```python
from build123d import *

# Parameters (mm, degrees)
SKETCH1_W           = 170
SKETCH1_H           = 120
BOSS_EXTRUDE1_DEPTH = 8
SKETCH2_W           = 41.380626675
SKETCH2_H           = 10
BOSS_EXTRUDE2_DEPTH = 8
SKETCH3_R           = 2
CUT_EXTRUDE1_DEPTH  = 8


with BuildPart() as part:
    # Sketch1 → Boss-Extrude1 (new body)
    with BuildSketch(Plane(origin=(0, 0, 0), x_dir=(1, 0, 0), z_dir=(0, 1, 0))):
        Rectangle(SKETCH1_W, SKETCH1_H)
    extrude(amount=BOSS_EXTRUDE1_DEPTH)

    # Sketch2 → Boss-Extrude2 (add)
    with BuildSketch(Plane(origin=(-17.791513114, 8, -1.374929401), x_dir=(1, 0, 0), z_dir=(0, 1, 0))):
        with Locations((-32.208486886, 28.840032215)):
            Rectangle(SKETCH2_W, SKETCH2_H)
    extrude(amount=BOSS_EXTRUDE2_DEPTH)

    # Sketch3 → Cut-Extrude1 (cut)
    with BuildSketch(Plane(origin=(0, 8, 0), x_dir=(1, 0, 0), z_dir=(0, 1, 0))):
        with Locations((-80, 55)):
            Circle(SKETCH3_R)
        with Locations((-80, -55)):
            Circle(SKETCH3_R)
        with Locations((80, 55)):
            Circle(SKETCH3_R)
        with Locations((80, -55)):
            Circle(SKETCH3_R)
    extrude(amount=-CUT_EXTRUDE1_DEPTH, mode=Mode.SUBTRACT)


solid = part.part
```
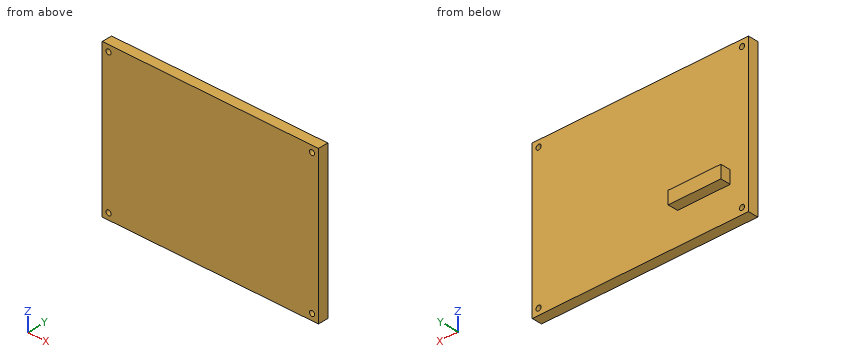
Read the model definition and answer for the solid it produces. Units are mm, in the model's axes. Give positions to 0.01 mm unless a question says otherwise; leave off trailing zeros. Write each loop counter-clockwise with the first axis right and the second up, starting at its lowest first coordinate (ties: lowest second). Pieces come first, ordered by that corner, then holes. Notation, with made-up numbers: M 66,27.25 L 95,27.25 A28 ccw 95,48.25 Z; hole C 51.5,-27.75 d2. An arc over 180 degrees is marked long. Put each result on its own line as item: value. Start each with the question number.
1. The part is cut by section D-D, the plane y = 12. Give the vertices of the cut face in (x, z).
2. The part is cut by section A-A, the plane x = -80. Give the vertices of the cut face in (y, z), and give its area (3 significant figures).
3. The part is cut by section B-B, the plane z = -55. Give the vertices of the cut face in (x, y), and give its area (3 significant figures).
4. The part is cut by section C-C, the plane x = -42.5. Give the vertices of the cut face in (y, z).
5. Consider line 1 along Z through (x, y) = (-80, 2.25); line 2 along X through (y, z) = (4.75, 55); line 3 along Y through (x, z) = (53.5, 52.5). Determine where each line is inside the solid, lowest interval first.
6. Each of these flat-tipped pins is pushed along its axis until it touches: pin 1 Ø3 at (x, z) = (80, 55) entering from +Y; pin 2 Ø4 at (y, z) = (12, -29.5) entering from +X; pin 3 Ø2.5 at (x, y) = (-42, 12.5) entering from +Z; pin 4 Ø6.5 at (x, z) = (-80, 55) entering from +Y. Where does it stop, or does it pass through?
Final values:
1. outline: M -70.69,-35.21 L -29.31,-35.21 L -29.31,-25.21 L -70.69,-25.21 Z
2. outline: M 0,-60 L 8,-60 L 8,-57 L 0,-57 Z; M 0,-53 L 8,-53 L 8,53 L 0,53 Z; M 0,57 L 8,57 L 8,60 L 0,60 Z
2. area: 896 mm²
3. outline: M -85,0 L -82,0 L -82,8 L -85,8 Z; M -78,0 L 78,0 L 78,8 L -78,8 Z; M 82,0 L 85,0 L 85,8 L 82,8 Z
3. area: 1,300 mm²
4. outline: M 0,-60 L 8,-60 L 8,-35.21 L 16,-35.21 L 16,-25.21 L 8,-25.21 L 8,60 L 0,60 Z
5. line 1: z = -60 to -57, -53 to 53, 57 to 60
5. line 2: x = -85 to -82, -78 to 78, 82 to 85
5. line 3: y = 0 to 8
6. pin 1: passes through
6. pin 2: stops at x = -29.31
6. pin 3: stops at z = -25.21
6. pin 4: stops at y = 8
